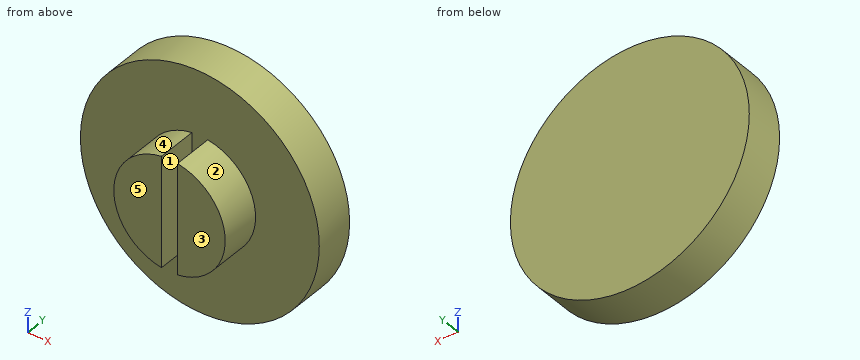
```python
from build123d import *

# Parameters (mm, degrees)
F0_R     = 19.05
F1_DEPTH = 6.35
F3_DEPTH = 38.1
F4_DEPTH = 25.4


with BuildPart() as f1:
    # F0 (on Front) → F1 (new body)
    with BuildSketch(Plane.XZ):
        Circle(F0_R)
    extrude(amount=F1_DEPTH)

    # F2 (on Front) → F3 (join)
    with BuildSketch(Plane.XZ):
        with BuildLine():
            Line((-1.27, -8.798818), (-1.27, 8.798818))
            ThreePointArc((-1.27, 8.798818), (-8.89, 0), (-1.27, -8.798818))
        make_face()
        with BuildLine():
            ThreePointArc((1.27, -8.798818), (8.89, 0), (1.27, 8.798818))
            Line((1.27, 8.798818), (1.27, -8.798818))
        make_face()
    extrude(amount=F3_DEPTH)

    # F3_face (on face) → F4 (cut)
    with BuildSketch(Plane(origin=(4.46805, -38.1, 0), x_dir=(1, 0, 0), z_dir=(0, -1, 0))):
        with BuildLine():
            Line((-3.19805, 8.798818), (-3.19805, -8.798818))
            ThreePointArc((-3.19805, -8.798818), (4.42195, 0), (-3.19805, 8.798818))
        make_face()
        with BuildLine():
            Line((-5.73805, -8.798818), (-5.73805, 8.798818))
            ThreePointArc((-5.73805, 8.798818), (-13.35805, 0), (-5.73805, -8.798818))
        make_face()
    extrude(amount=-F4_DEPTH, mode=Mode.SUBTRACT)


solid = f1.part
```
Can you work these out from the model? Positions are in its coordinate system, mm. Face numbers are marked on the shaded views. A direction names the side the tool comes from. Coordinates: 2 decimals unless noted, no trailing zeros. Order: outer loops, then holes, each group sorted by start corner. A loop starts at its lowest first (then second) coordinate and runs counter-clockwise, first axis right, second up.
1. I need wall thicknesses on line 1 (X direction, y = -7.5, z = 0); line 2 (Y direction, x = 10, z = 8); line 3 (X direction, y = -11.25, z = 7). Which ranges of each line are inside material? Lowest first, please.
2. If we section it at A-A (z = 0): Please give me the cut outline in (x, y).
3. For the marked faces 4 and 5, which set-ups out of +Z, -Z, +X, -X, +Y, -Y let a thin tool reach every point of the face, with its end or its side?
4. If we section it at D-D (y = -3.75): Please give me the cut outline in (x, z), then the cut area to 3 significant figures.
5. I'm going to push flat-ended pins straight in: pin 1 (1.9 mm diameter, centred on y = -10, z = 0, fed in from -X); pin 2 (1 mm diameter, centred on y = -7.5, z = 6, fed in from -X); pin 3 (6 mm diameter, centred on x = -12.5, y = -10, fed in from -Z); pin 4 (1.5 mm diameter, centred on y = -6, z = -6.5, fed in from -X). Where does each tip first touch, or does it pass through?
6. Thinking about a two-plate mould opening in X: for the marked faces 1, 2 and 3, which applies, +X half, -X half, draft (parallel to the pull), parting line (faces both ways), or undercut?
7. If we section it at B-B (x = 2): Please give me the cut outline in (y, z), then the cut area to 3 significant figures.
8. If we section it at C-C (y = -7.5): Please give me the cut outline in (x, z), then the cut area to 3 significant figures.
Entries:
1. line 1: x = -8.89 to -1.27, 1.27 to 8.89
1. line 2: y = -6.35 to 0
1. line 3: x = -5.48 to -1.27, 1.27 to 5.48
2. outline: (-19.05, -6.35) - (-8.89, -6.35) - (-8.89, -12.7) - (-1.27, -12.7) - (-1.27, -6.35) - (1.27, -6.35) - (1.27, -12.7) - (8.89, -12.7) - (8.89, -6.35) - (19.05, -6.35) - (19.05, 0) - (-19.05, 0) - close
3. face 4: -X, -Y
3. face 5: +Z, -Z, +X, -X, -Y
4. outline: circle Ø38.1 at (0, 0)
4. area: 1,140 mm2
5. pin 1: stops at x = -8.89
5. pin 2: stops at x = -6.98
5. pin 3: passes through
5. pin 4: stops at x = -18.16
6. face 1: undercut
6. face 2: +X half
6. face 3: draft
7. outline: (-12.7, -8.66) - (-6.35, -8.66) - (-6.35, -18.94) - (0, -18.94) - (0, 18.94) - (-6.35, 18.94) - (-6.35, 8.66) - (-12.7, 8.66) - close
7. area: 351 mm2
8. outline: (-1.27, -8.8) - (-1.27, 8.8) arc R8.89 ccw to start; (1.27, -8.8) arc R8.89 ccw to (1.27, 8.8) - close
8. area: 203 mm2
